from build123d import *

# Parameters (mm, degrees)
F0_R     = 38.1
F0_R_2   = 20.701
F1_DEPTH = 38.1
F2_R     = 3.175
F3_R     = 3.302
F4_DEPTH = 50.8
F3_R_2   = 4.064
F5_DEPTH = 33.528
F3_R_3   = 5.08
F6_DEPTH = 21.844
F7_R     = 1.6002


with BuildPart() as f1:
    # F0 (on Front) → F1 (new body)
    with BuildSketch(Plane.XZ):
        Circle(F0_R)
        Circle(F0_R_2, mode=Mode.SUBTRACT)
    extrude(amount=F1_DEPTH)

    # F2
    f2_edges = [f1.edges().sort_by_distance(p)[0] for p in [
        (-38.1, -38.1, 0),
    ]]
    fillet(f2_edges, radius=F2_R)

    # F3 (on Right) → F4 (cut, symmetric)
    with BuildSketch(Plane.YZ):
        with Locations((-9.406389, 0)):
            Circle(F3_R)
    extrude(amount=F4_DEPTH, both=True, mode=Mode.SUBTRACT)

    # F3 (on Right) → F5 (cut, symmetric)
    with BuildSketch(Plane.YZ):
        with Locations((-9.406389, 0)):
            Circle(F3_R_2)
        with Locations((-9.406389, 0)):
            Circle(F3_R, mode=Mode.SUBTRACT)
    extrude(amount=F5_DEPTH, both=True, mode=Mode.SUBTRACT)

    # F3 (on Right) → F6 (cut, symmetric)
    with BuildSketch(Plane.YZ):
        with Locations((-9.406389, 0)):
            Circle(F3_R_3)
        with Locations((-9.406389, 0)):
            Circle(F3_R_2, mode=Mode.SUBTRACT)
    extrude(amount=F6_DEPTH, both=True, mode=Mode.SUBTRACT)

    # F7
    f7_edges = [f1.edges().sort_by_distance(p)[0] for p in [
        (-20.701, -38.1, 0),
        (-20.701, 0, 0),
    ]]
    fillet(f7_edges, radius=F7_R)


solid = f1.part
Design review of the part built by this model. Coordinates are the model's own, in mm. A direction names the side the tool comes from. Round coordinates to 2 decimals unless told otherwise and drop trailing zeros. Write each loop counter-clockwise with the first axis right and the second up, starting at its lowest first coordinate (ties: lowest second). Pieces come first, ordered by that corner, then holes. Notation, with made-up numbers: M -9,25 L 38,25 A25 ccw 38,60 Z; hole C 6,-3.5 d8. An arc over 180 degrees is marked long. One line per item, written item: value. Start each with the question number.
1. Take a section at C-C on z = 0. State how many separate pieces and enclosed holes the cut face has, then the cut area to 3 significant figures.
2. Take a section at D-D on y = -22.5. State the section outline as (x, z) points, then the cut area to 3 significant figures.
3. To check wall thickness, follow probe 1 along Z at (x, y) = (11, -34); probe 2 along X at (y, z) = (-29, 2.5); probe 3 along Z at (x, y) = (0, -24). State the ranges of each line that lie inside material, in increasing order. Write a range as from..to.
4. For faces 1 (the face through (36.34, -17.22, 11.44)), 2 (the face through (21.17, -14.48, 0.22)), list the 3-axis set-ups (+Z, -Z, +X, -X, +Y, -Y) from which the entire face can be reached by the end or side of a thin tool; tool diameter is ignored.
5. Clearance check with flat-ended pins moving along their axes: P1, Ø5, axis at y = -9.41, z = 0, coming from the +X side; P2, Ø3, axis at y = -9.5, z = 2.5, coming from the +X side; P3, Ø10, axis at y = -7.5, z = -6, coming from the -X side; P4, Ø2.5, axis at y = -11.5, z = -1.5, coming from the +X side. State where each tip first meets the part, or that it passes through.
6. Take a section at B-B on y = -9. State the section outline as (x, z) points, then the cut area to 3 significant figures.
7. Take a section at A-A on x = 0. State the section outline as (y, z) points (3 decimals).
8. Draft analysis for pull direction Y (two halves, no side actions). For faces 3 (the face through (16, 0, -16)), 4 (the face through (0, -38.1, -23)), 5 (the face through (-21.844, -8, 4)), state which applies: pulls with the +Y half, pulls with the -Y half, needs draft (parallel to the pull), parting line crosses it, or undercut.
Computed:
1. separate pieces: 4
1. enclosed holes: 0
1. area: 1,050 mm²
2. outline: C 0,0 d76.2; hole C 0,0 d41.4
2. area: 3,210 mm²
3. probe 1: z = -36.48..-17.54, 17.54..36.48
3. probe 2: x = -38.02..-20.55, 20.55..38.02
3. probe 3: z = -38.1..-20.7, 20.7..38.1
4. face 1: +Y, -Y
4. face 2: none
5. P1: passes through
5. P2: stops at x = 37.99
5. P3: stops at x = -38.08
5. P4: stops at x = 38.09
6. outline: M -37.96,-3.28 A38.1 ccw 37.96,-3.28 L 33.53,-3.28 L 33.53,-4.04 L 21.84,-4.04 L 21.84,-5.06 L 20.07,-5.06 A20.7 cw -20.07,-5.06 L -21.84,-5.06 L -21.84,-4.04 L -33.53,-4.04 L -33.53,-3.28 Z; M -37.96,3.28 L -33.53,3.28 L -33.53,4.04 L -21.84,4.04 L -21.84,5.06 L -20.07,5.06 A20.7 cw 20.07,5.06 L 21.84,5.06 L 21.84,4.04 L 33.53,4.04 L 33.53,3.28 L 37.96,3.28 A38.1 ccw Z
6. area: 2,940 mm²
7. outline: M -38.1,-34.925 A3.175 ccw -34.925,-38.1 L 0,-38.1 L 0,-22.301 A1.6 ccw -1.6,-20.701 L -36.5,-20.701 A1.6 ccw -38.1,-22.301 Z; M -38.1,22.301 A1.6 ccw -36.5,20.701 L -1.6,20.701 A1.6 ccw 0,22.301 L 0,38.1 L -34.925,38.1 A3.175 ccw -38.1,34.925 Z
8. face 3: pulls with the +Y half
8. face 4: pulls with the -Y half
8. face 5: undercut
